from build123d import *


with BuildPart() as part:
    # Эскиз1 → Повернуть1 (revolve)
    with BuildSketch(Plane.XY, mode=Mode.PRIVATE) as revolve_1_sk:
        with BuildLine():
            Line((0, 7.25), (0, 5.25))
            Line((0, 5.25), (9, 5.25))
            Line((9, 5.25), (10, 4.25))
            Line((10, 4.25), (18.75, 4.25))
            Line((18.75, 4.25), (19.5, 5))
            Line((19.5, 5), (19.5, 5.7))
            Line((19.5, 5.7), (18.75, 6.45))
            Line((18.75, 6.45), (6.7, 6.45))
            ThreePointArc((6.7, 6.45), (5.1, 8.05), (3.5, 6.45))
            Line((3.5, 6.45), (1, 6.45))
            Line((1, 6.45), (0, 7.25))
        make_face()
    revolve(revolve_1_sk.sketch.rotate(Axis((0, 0, 0), (-1, 0, 0)), 90), axis=Axis((0, 0, 0), (-1, 0, 0)))


solid = part.part
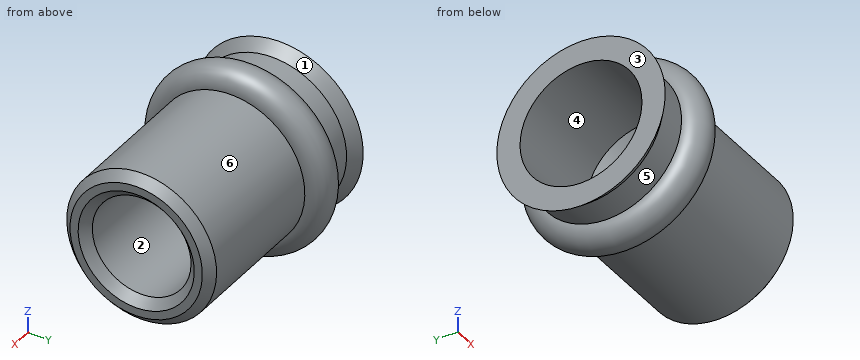
Design review of the part built by this model. Coordinates are the model's own, in mm. Face numbers are marked on the shaded views. A direction names the side the tool comes from. Give positions to 0.01 mm unless a question says otherwise; leave off trailing zeros. Write each loop counter-clockwise with the first axis right and the second up, starting at its lowest first coordinate (ties: lowest second). Pieces come first, ordered by that corner, then holes. Notation, with made-up numbers: M 43.5,-14.5 L 67.5,-14.5 A11 ccw 67.5,-10.5 Z; hole C 42.5,-31 d5. An arc over 180 degrees is marked long. Return JSON: item names as keys, results as strings. Group by question number.
Item 1: Take a section at D-D (x = 17.25). Give the boundary of the cut face in (y, z), plus the area to 3 significant figures.
Item 2: Take a section at C-C (x = 9.25). Give the boundary of the cut face in (y, z), plus the area to 3 significant figures.
Item 3: The part is to be moulded in two halves that separate along X. For the marked faces 1, 2 and 3, say which applies: pulls with the +X half, pulls with the -X half, needs draft (parallel to the pull), parting line crosses it, or undercut.
Item 4: Wall thickness on line 1 along Y through (x, z) = (5, 0); line 2 along Z through (x, y) = (8, -0.25); line 3 along Y through (x, z) = (16.75, 0): over which ranges is each line inside the solid? List them lowest first.
Item 5: Tool access review of the marked faces 4, 5 and 6: name each direction out of +Z, -Z, +X, -X, +Y, -Y from which nothing blocks a thin tool from reaching the whole face with its end or side.
Item 6: Take a section at A-A (z = 0). Give the boundary of the cut face in (x, y), plus the area to 3 significant figures.
Item 7: Clearance check with flat-ended pins moving along their axes: pin 1 Ø1 at (x, y) = (14, 5) entering from -Z; pin 2 Ø2 at (x, y) = (16.5, -4.5) entering from -Z; pin 3 Ø2 at (x, z) = (11.5, 2.5) entering from -Y. State where each tip first meets the part, or that it passes through.
Return value:
{
 "1": {"outline": "C 0,0 d12.9; hole C 0,0 d8.5", "area": "74.0 mm2"},
 "2": {"outline": "C 0,0 d12.9; hole C 0,0 d10", "area": "52.2 mm2"},
 "3": {"face 1": "undercut", "face 2": "needs draft", "face 3": "pulls with the -X half"},
 "4": {"line 1": "y = -8.05 to -5.25, 5.25 to 8.05", "line 2": "z = -6.45 to -5.24, 5.24 to 6.45", "line 3": "y = -6.45 to -4.25, 4.25 to 6.45"},
 "5": {"face 4": "-X", "face 5": "none", "face 6": "+X"},
 "6": {"outline": "M 0,-7.25 L 1,-6.45 L 3.5,-6.45 A1.6 ccw 6.7,-6.45 L 18.75,-6.45 L 19.5,-5.7 L 19.5,-5 L 18.75,-4.25 L 10,-4.25 L 9,-5.25 L 0,-5.25 Z; M 0,5.25 L 9,5.25 L 10,4.25 L 18.75,4.25 L 19.5,5 L 19.5,5.7 L 18.75,6.45 L 6.7,6.45 A1.6 ccw 3.5,6.45 L 1,6.45 L 0,7.25 Z", "area": "74.5 mm2"},
 "7": {"pin 1": "stops at z = -4.62", "pin 2": "stops at z = -5.42", "pin 3": "stops at y = -6.27"}
}
